Here's the drawing with two shaded views (mm, measured from the low corner). I have some questions. Coordinates: 2 decimals unless noted, no trailing zeros. Loops run counter-clockwise (first coordinate to the right, second up) from the corner with the lowest first, then second, coordinate; pieces in that order, holes last. Notation, with made-up numbers: (89.25, 23.5) -> (111.25, 23.5) arc R19 ccw to (111.25, 31.5) -> close; hole circle Ø8 at (83, 62). An arc over 180 degrees is marked (long way). Answer as a JSON object with one key per item and string values. Group by question number.
1) I want a section at C-C (x = 10.75). Write out the boundary of the cut face in (y, z) (1 decimal).
2) If we mould it in two halves opening along Z, with no side actions, what happens to the marked faces 1, 2 and 3? For each: +Z half, -Z half, draft (parallel to the pull), parting line (faces both ways), or undercut.
3) I'm going to push flat-ended pins straight in: pin 1 (2 mm diameter, centred on y = 4.5, z = 4.5, fed in from -X); pin 2 (2 mm diameter, centred on x = 4.5, z = 5, fed in from +Y); pin 3 (1.5 mm diameter, centred on y = 2.5, z = 6, fed in from +X). Where does each tip first touch, or does it pass through?
4) I need wall thicknesses on probe 1 along Z at (x, y) = (7, 1.3) (1 decimal); probe 2 along X at (y, z) = (2.6, 8.25) (1 decimal); probe 3 along Z at (x, y) = (6.25, 2) (1 decimal). Which ranges of each line are inside material? Lowest first, please. Write a range as [from, to].
5) I want a section at B-B (z = 9.5). Write out the boundary of the cut face in (x, y) (1 decimal).
6) I want a section at A-A (x = 6). Write out the boundary of the cut face in (y, z) (1 decimal), then the cut area to 3 significant figures.
7) I want a section at D-D (z = 2.25). Write out the boundary of the cut face in (x, y).
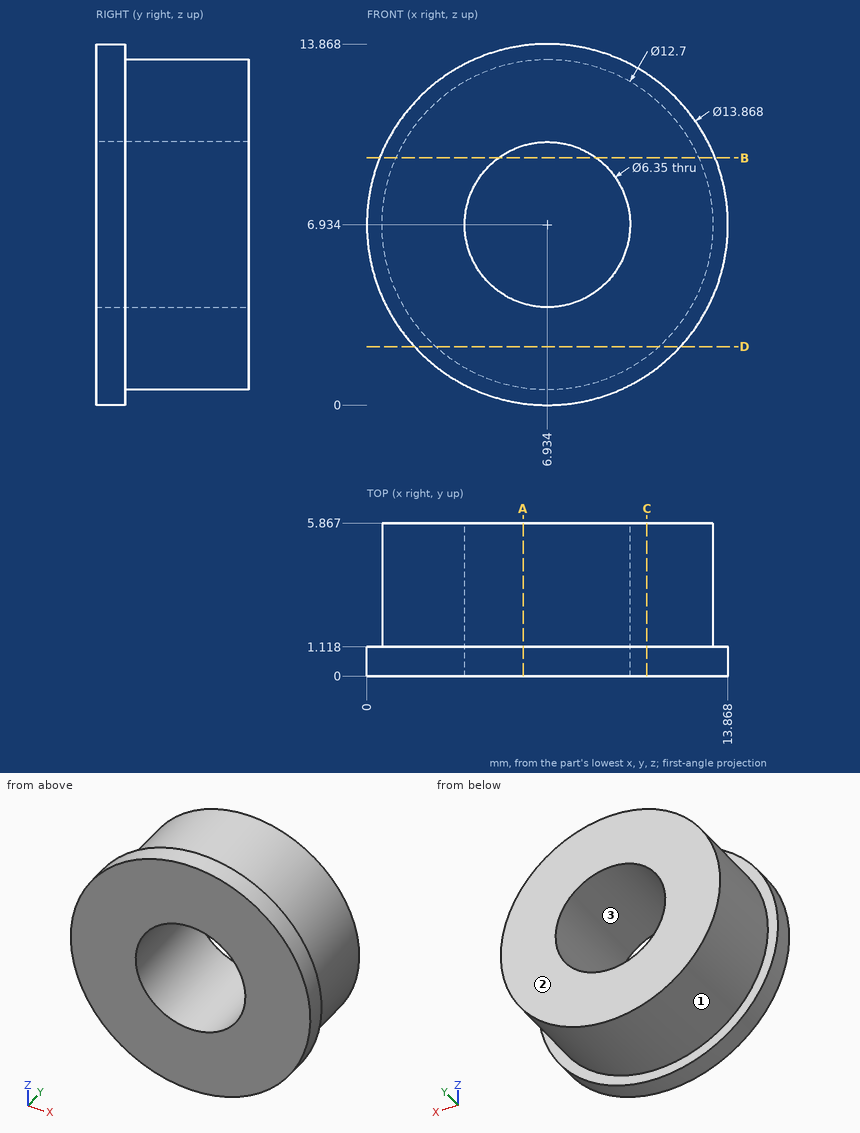
Determined:
{
 "1": {"outline": "(0, 1.1) -> (1.1, 1.1) -> (1.1, 1.9) -> (5.9, 1.9) -> (5.9, 12) -> (1.1, 12) -> (1.1, 12.7) -> (0, 12.7) -> close"},
 "2": {"face 1": "parting line", "face 2": "draft", "face 3": "undercut"},
 "3": {"pin 1": "x = 0.75", "pin 2": "y = 5.87", "pin 3": "x = 13.28"},
 "4": {"probe 1": "[0.6, 3.8], [10.1, 13.3]", "probe 2": "[0.7, 4], [9.8, 13.1]", "probe 3": "[0.6, 3.8], [10, 13.2]"},
 "5": {"outline": "(0.5, 0) -> (5.1, 0) -> (5.1, 5.9) -> (1.1, 5.9) -> (1.1, 1.1) -> (0.5, 1.1) -> close; (8.8, 0) -> (13.4, 0) -> (13.4, 1.1) -> (12.7, 1.1) -> (12.7, 5.9) -> (8.8, 5.9) -> close"},
 "6": {"outline": "(0, 0.1) -> (1.1, 0.1) -> (1.1, 0.7) -> (5.9, 0.7) -> (5.9, 3.9) -> (0, 3.9) -> close; (0, 10) -> (5.9, 10) -> (5.9, 13.2) -> (1.1, 13.2) -> (1.1, 13.8) -> (0, 13.8) -> close", "area": "39.4 mm^2"},
 "7": {"outline": "(1.82, 0) -> (12.05, 0) -> (12.05, 1.12) -> (11.22, 1.12) -> (11.22, 5.87) -> (2.65, 5.87) -> (2.65, 1.12) -> (1.82, 1.12) -> close"}
}
